The listing builds one solid part. Answer for the finished solid, in the listing's coordinates (mm). A direction names the side the tool comes from. Give positions to 0.01 mm unless a question says otherwise; leave off trailing zeros. Write each loop counter-clockwise with the first axis right and the second up, starting at its lowest first coordinate (ties: lowest second). Pieces come first, ordered by that corner, then holes. Notation, with made-up numbers: (-37, -4.5) - (-12, -4.5) arc R25 ccw to (-12, 17.5) - close; hole circle Ø7 at (55.5, -17.75). An arc over 180 degrees is marked (long way). Return JSON: item names as keys, results as strings.
from build123d import *

# Parameters (mm, degrees)
BOSS_EXTRUDE1_DEPTH = 4
SKETCH2_R           = 10
BOSS_EXTRUDE2_DEPTH = 4
SKETCH3_R           = 6
CUT_EXTRUDE1_DEPTH  = 81.443271937


with BuildPart() as part:
    # Sketch1 → Boss-Extrude1 (new body)
    with BuildSketch(Plane(origin=(0, 0, 0), x_dir=(1, 0, 0), z_dir=(0, 1, 0))):
        with BuildLine():
            Line((6, 56.6), (6, 17.1))
            ThreePointArc((6, 17.1), (0, 11.1), (-6, 17.1))
            Line((-6, 17.1), (-6, 56.6))
            Line((-6, 56.6), (-10.6, 56.6))
            ThreePointArc((-10.6, 56.6), (-24.073088065, 24.073088065), (-56.6, 10.6))
            Line((-56.6, 10.6), (-56.6, 6))
            Line((-56.6, 6), (-17.1, 6))
            ThreePointArc((-17.1, 6), (-11.1, 0), (-17.1, -6))
            Line((-17.1, -6), (-56.6, -6))
            Line((-56.6, -6), (-56.6, -10.6))
            ThreePointArc((-56.6, -10.6), (-24.073088065, -24.073088065), (-10.6, -56.6))
            Line((-10.6, -56.6), (-6, -56.6))
            Line((-6, -56.6), (-6, -17.1))
            ThreePointArc((-6, -17.1), (0, -11.1), (6, -17.1))
            Line((6, -17.1), (6, -56.6))
            Line((6, -56.6), (10.6, -56.6))
            ThreePointArc((10.6, -56.6), (24.073088065, -24.073088065), (56.6, -10.6))
            Line((56.6, -10.6), (56.6, -6))
            Line((56.6, -6), (17.1, -6))
            ThreePointArc((17.1, -6), (11.1, 0), (17.1, 6))
            Line((17.1, 6), (56.6, 6))
            Line((56.6, 6), (56.6, 10.6))
            ThreePointArc((56.6, 10.6), (24.073088065, 24.073088065), (10.6, 56.6))
            Line((10.6, 56.6), (6, 56.6))
        make_face()
    extrude(amount=BOSS_EXTRUDE1_DEPTH)

    # Sketch2 → Boss-Extrude2 (add)
    with BuildSketch(Plane(origin=(0, 4, 0), x_dir=(1, 0, 0), z_dir=(0, 1, 0))):
        with Locations(Location((0, 0, 0), (0, 0, 270))):
            Circle(SKETCH2_R)
    extrude(amount=BOSS_EXTRUDE2_DEPTH)

    # Sketch3 → Cut-Extrude1 (cut, through all)
    with BuildSketch(Plane(origin=(0, 8, 0), x_dir=(1, 0, 0), z_dir=(0, 1, 0))):
        with Locations(Location((0, 0, 0), (0, 0, 270))):
            Circle(SKETCH3_R)
    extrude(amount=-CUT_EXTRUDE1_DEPTH, mode=Mode.SUBTRACT)


solid = part.part
Item 1: A cutting plane is placed at B-B on z = -19. Determine the outline of the cut face in (x, y).
Answer below:
{"outline": "(-30.1, 0) - (-6, 0) - (-6, 4) - (-30.1, 4) - close; (6, 0) - (30.1, 0) - (30.1, 4) - (6, 4) - close"}
Item 2: A cutting plane is placed at D-D on x = -29.5. Determine the outline of the cut face in (y, z), then the cut area to 3 significant figures.
Answer below:
{"outline": "(0, -19.43) - (4, -19.43) - (4, -6) - (0, -6) - close; (0, 6) - (4, 6) - (4, 19.43) - (0, 19.43) - close", "area": "107 mm²"}
Item 3: Consider L1, parallel to X at y = 2, z = 0; L2, parallel to Y at x = -8.5, z = 28.5; L3, parallel to X at y = 6.25, z = 0. Determine where each line is inside the solid, lowest interval first.
Answer below:
{"L1": "x = -11.1 to -6, 6 to 11.1", "L2": "y = 0 to 4", "L3": "x = -10 to -6, 6 to 10"}
Item 4: A cutting plane is placed at A-A on x = 0. Determine the outline of the cut face in (y, z).
Answer below:
{"outline": "(0, -11.1) - (4, -11.1) - (4, -10) - (8, -10) - (8, -6) - (0, -6) - close; (0, 6) - (8, 6) - (8, 10) - (4, 10) - (4, 11.1) - (0, 11.1) - close"}
Item 5: Flat-ended cylindrical pins translate along their axes: P1, Ø4.5, axis at x = -29, y = 2, coming from the +Z side; P2, Ø1.2, axis at y = 1, z = -38, coming from the +X side; P3, Ø2, axis at x = -43, y = 2, coming from the -Z side. Find the tip coordinate at first contact, or state that the pin passes through.
Answer below:
{"P1": "stops at z = 21.6", "P2": "stops at x = 14.8", "P3": "stops at z = -12.98"}
Item 6: The mould has two halves that part along Z. Classify faces 1 (the face through (1.802, 4.056, 5.723)), 2 (the face through (6, 2, 37)), 3 (the face through (23.72, 1.97, 24.43)), 4 (the face through (37, 2, -6)): +Z half, -Z half, draft (parallel to the pull), parting line (faces both ways), or undercut.
Answer below:
{"face 1": "undercut", "face 2": "draft", "face 3": "+Z half", "face 4": "undercut"}
Item 7: A cutting plane is placed at C-C on y = 6.25. Determine the outline of the cut face in (x, z).
Answer below:
{"outline": "circle Ø20 at (0, 0); hole circle Ø12 at (0, 0)"}
Item 8: For faces 5 (the face through (-6, 2, 37)), 6 (the face through (37, 2, 6)), 7 (the face through (-37, 2, 6)), 8 (the face through (-6, 2, -37)), 9 (the face through (-9, 4, 8)), determine the directions among +Z, -Z, +X, -X, +Y, -Y from which every point of the face is accessible in a straight line to the end or side of a thin tool.
Answer below:
{"face 5": "+Z, +Y, -Y", "face 6": "+X, +Y, -Y", "face 7": "-X, +Y, -Y", "face 8": "-Z, +Y, -Y", "face 9": "+Y"}
